Read the model definition and answer for the solid it produces. Units are mm, in the model's axes. A direction names the side the tool comes from. Give positions to 0.01 mm unless a question says otherwise; leave off trailing zeros. Order: outer loops, then holes, each group sorted by start corner. A loop starts at its lowest first (then second) coordinate and runs counter-clockwise, first axis right, second up.
Item 1: Find the intervals of material crossed by line 1 along Z through (x, y) = (11.15, 3.4); line 2 along X through (y, z) = (2.25, 11.7); line 3 along X through (y, z) = (2, 22), in increasing order.
Item 2: A cutting plane is placed at A-A (z = 11.7). Write down the section's boundary in (x, y), plus the area to 3 significant figures.
Item 3: A cutting plane is placed at C-C (y = 13.5). Write down the section's boundary in (x, z), plus the area to 3 significant figures.
Item 4: A cutting plane is placed at B-B (x = -11.15). Write down the section's boundary in (y, z).
Item 5: The mould has two halves that part along X. Classify faces 1 (the face through (-2, -6, -25)), 2 (the face through (-15, 10, 0)), 3 (the face through (-18, 8, 0)): +X half, -X half, draft (parallel to the pull), parting line (faces both ways), or undercut.
Item 6: Which of the six approach directions +Z, -Z, +X, -X, +Y, -Y give full straight-line access (tool end or side, diameter ignored) to faces 4 (the face through (5.5, 10, 0)), 5 (the face through (12, 5, 0)), 6 (the face through (-5, -15, -28)), 7 (the face through (-7.425, -5, -28))?
Item 7: Given pin 1 Ø3 at (x, z) = (5, -4.5) entering from -Y; pin 2 Ø3 at (y, z) = (-9.5, -28.5) entering from -X (3 decimals); pin 3 Ø16 at (x, y) = (-6.5, -9) entering from +Z, each flat-ended and moving along its own axis, determine where each tip first touches the part or whether it passes through.
Item 8: A cutting plane is placed at D-D (x = 13.5). Write down the section's boundary in (y, z), plus the area to 3 significant figures.
from build123d import *

# Parameters (mm, degrees)
SKETCH_1_W               = 30
SKETCH_1_H               = 50
EXTRUDE_1_DEPTH          = 5
SKETCH_2_R               = 1.5
CUT_EXTRUDE_2_DEPTH      = 6
CUT_EXTRUDE_2_DEPTH_BACK = 3
SKETCH_3_W               = 30
SKETCH_3_H               = 25
EXTRUDE_2_DEPTH          = 3
SKETCH_4_W               = 4.85
SKETCH_4_H               = 20
EXTRUDE_3_DEPTH          = 6
EXTRUDE_START            = -50
SKETCH_6_W               = 3
SKETCH_6_H               = 16
EXTRUDE_4_DEPTH          = 50


with BuildPart() as part:
    # 스케치1 → 보스-돌출1 (new body)
    with BuildSketch(Plane(origin=(0, 0, 0), x_dir=(1, 0, 0), z_dir=(0, 1, 0))):
        Rectangle(SKETCH_1_W, SKETCH_1_H)
    extrude(amount=EXTRUDE_1_DEPTH)

    # 스케치2 → 컷-돌출2 (cut, two sides)
    with BuildSketch(Plane(origin=(0, 0, 0), x_dir=(1, 0, 0), z_dir=(0, 1, 0))) as cut_extrude_2_sk:
        with Locations((-11.15, -11.7)):
            Circle(SKETCH_2_R)
        with Locations((11.15, -22)):
            Circle(SKETCH_2_R)
    extrude(amount=CUT_EXTRUDE_2_DEPTH, mode=Mode.SUBTRACT)
    extrude(cut_extrude_2_sk.sketch, amount=-CUT_EXTRUDE_2_DEPTH_BACK, mode=Mode.SUBTRACT)

    # 스케치3 → 보스-돌출2 (add)
    with BuildSketch(Plane(origin=(0, 0, -25), x_dir=(-1, 0, 0), z_dir=(0, 0, -1))):
        with Locations((0, -7.5)):
            Rectangle(SKETCH_3_W, SKETCH_3_H)
    extrude(amount=-EXTRUDE_2_DEPTH)

    # 스케치4 → 보스-돌출3 (add)
    with BuildSketch(Plane(origin=(0, 0, -25), x_dir=(-1, 0, 0), z_dir=(0, 0, -1))):
        with Locations((5, -5)):
            Rectangle(SKETCH_4_W, SKETCH_4_H)
    extrude(amount=EXTRUDE_3_DEPTH)

    # 스케치6 → 보스-돌출4 (add)
    with BuildSketch(Plane.XY.offset(25).offset(EXTRUDE_START)):
        with Locations((-16.5, 8)):
            Rectangle(SKETCH_6_W, SKETCH_6_H)
        with Locations((7, 8)):
            Rectangle(SKETCH_6_W, SKETCH_6_H)
    extrude(amount=EXTRUDE_4_DEPTH)


solid = part.part
Response values:
1. line 1: z = -25 to 20.5, 23.5 to 25
1. line 2: x = -18 to -12.65, -9.65 to 15
1. line 3: x = -18 to 9.65, 12.65 to 15
2. outline: (-18, 0) - (-12.65, 0) - (-12.65, 5) - (-15, 5) - (-15, 16) - (-18, 16) - close; (-9.65, 0) - (15, 0) - (15, 5) - (8.5, 5) - (8.5, 16) - (5.5, 16) - (5.5, 5) - (-9.65, 5) - close
2. area: 216 mm2
3. outline: (-18, -25) - (-15, -25) - (-15, 25) - (-18, 25) - close; (5.5, -25) - (8.5, -25) - (8.5, 25) - (5.5, 25) - close
3. area: 300 mm2
4. outline: (-20, -25) - (5, -25) - (5, 10.2) - (0, 10.2) - (0, -22) - (-20, -22) - close; (0, 13.2) - (5, 13.2) - (5, 25) - (0, 25) - close
5. face 1: draft
5. face 2: undercut
5. face 3: -X half
6. face 4: +Z, -Z, +Y
6. face 5: +Z, -Z, +X, +Y
6. face 6: -Z, +X, -X, -Y
6. face 7: -Z, -X, +Y, -Y
7. pin 1: stops at y = 0
7. pin 2: stops at x = -7.425
7. pin 3: stops at z = -22
8. outline: (-20, -25) - (5, -25) - (5, 25) - (0, 25) - (0, -22) - (-20, -22) - close
8. area: 310 mm2
